from build123d import *

# Parameters (mm, degrees)
SKETCH1_W           = 4
SKETCH1_H           = 15
BOSS_EXTRUDE1_DEPTH = 4
SKETCH2_R           = 0.925
BOSS_EXTRUDE2_DEPTH = 2
BOSS_EXTRUDE3_DEPTH = 2
SKETCH6_W           = 5
SKETCH6_H           = 5
BOSS_EXTRUDE5_DEPTH = 7.5
SKETCH7_R           = 0.925
BOSS_EXTRUDE6_DEPTH = 18
CHAMFER1_SIZE       = 0.5


with BuildPart() as part:
    # Sketch1 → Boss-Extrude1 (new body)
    with BuildSketch(Plane(origin=(0, 0, 0), x_dir=(1, 0, 0), z_dir=(0, 1, 0))):
        Rectangle(SKETCH1_W, SKETCH1_H)
    extrude(amount=BOSS_EXTRUDE1_DEPTH)

    # Sketch2 → Boss-Extrude2 (add)
    with BuildSketch(Plane.XY.offset(7.5)):
        with Locations((0, 2)):
            Circle(SKETCH2_R)
    extrude(amount=BOSS_EXTRUDE2_DEPTH)

    # Sketch3 → Boss-Extrude3 (add)
    with BuildSketch(Plane.XY.offset(9.5)):
        with BuildLine():
            Line((-0.75, 2.925), (0.75, 2.925))
            ThreePointArc((0.75, 2.925), (1.675, 2), (0.75, 1.075))
            Line((0.75, 1.075), (-0.75, 1.075))
            ThreePointArc((-0.75, 1.075), (-1.675, 2), (-0.75, 2.925))
        make_face()
    extrude(amount=BOSS_EXTRUDE3_DEPTH)

    # Sketch6 → Boss-Extrude5 (add)
    with BuildSketch(Plane.XY):
        with Locations((0.5, 2.5)):
            Rectangle(SKETCH6_W, SKETCH6_H)
    extrude(amount=-BOSS_EXTRUDE5_DEPTH)

    # Sketch7 → Boss-Extrude6 (add)
    with BuildSketch(Plane.XY.offset(7.5)):
        with Locations((1, 2.832903413)):
            Circle(SKETCH7_R)
    extrude(amount=-BOSS_EXTRUDE6_DEPTH)

    # Chamfer1
    chamfer1_edges = [part.edges().sort_by_distance(p)[0] for p in [
        (-2, 4, 3.75),
        (3, 0, -3.75),
        (-2, 5, -3.75),
        (3, 5, -3.75),
        (2, 4, 3.75),
        (-2, 0, 0),
        (2, 0, 3.75),
    ]]
    chamfer(chamfer1_edges, length=CHAMFER1_SIZE)


solid = part.part
Verification items for the finished model (mm, model axes). A direction names the side the tool comes from. Coordinates: 2 decimals unless noted, no trailing zeros. Order: outer loops, then holes, each group sorted by start corner. A loop starts at its lowest first (then second) coordinate and runs counter-clockwise, first axis right, second up. Notation, with made-up numbers: M 4.25,-3.75 L 21.25,-3.75 A21 ccw 21.25,4.25 Z; hole C 72,49.25 d6. An arc over 180 degrees is marked long. One line per item, written item: value. Start each with the question number.
Item 1: Sectioned sample at B-B (x = 1.25). Enter the section's corners in (y, z), then the cut area to 3 significant figures.
Item 2: Sectioned sample at D-D (y = 1.35). Enter the section's corners in (x, z).
Item 3: Scan lines: probe 1 along Z at (x, y) = (1.05, 2.65); probe 2 along Y at (x, z) = (-0.45, 7.25); probe 3 along Z at (x, y) = (0.65, 0.75). Record each from-to range of solid material in increasing order.
Item 4: Mould release check, pull along Z, two halves, no side actions. Record for faces 5 (the flat face through (0, 2, -7.5)), 6 (the flat face through (0, 1.075, 10)), 7 (the flat face through (-1.2, 2, 9.5)): released by +Z, released by -Z, zero draft, split by the parting line, or undercut.
Item 5: Gauge pin test, flat ends, axial feed: pin 1 (1.6 mm diameter, centred on x = 0, z = 10.5, fed in from +Y) (3 decimals); pin 2 (0.8 mm diameter, centred on x = -1, y = 2, fed in from -Z); pin 3 (0.9 mm diameter, centred on x = 0, z = 4.5, fed in from +Y). Record the tip position at first contact, or that the pin passes through.
Item 6: Sectioned sample at C-C (x = 2.25). Enter the section's corners in (y, z).
Item 7: Sectioned sample at A-A (z = -2.5). Enter the section's corners in (x, y).
Item 8: Access from +Z, -Z, +X, -X, +Y, -Y to the whole of each face (thin tool, end or side, straight path). Record for faces 1 (the flat face through (2, 2, 4)), 2 (the flat face through (0, 2.925, 10)), 3 (the cylindrical face through (1.675, 2.02, 10.486)), 4 (the cylindrical face through (-1.675, 1.98, 10.486)).
Conclusion:
1. outline: M 0,-7.5 L 1.94,-7.5 L 1.94,-10.5 L 3.72,-10.5 L 3.72,-7.5 L 5,-7.5 L 5,0 L 4,0 L 4,7.5 L 0,7.5 Z; M 1.22,9.5 L 2.78,9.5 L 2.78,11.5 L 1.22,11.5 Z
1. area: 76.0 mm^2
2. outline: M -2,-7.5 L 3,-7.5 L 3,0 L 2,0 L 2,7.5 L 0.66,7.5 L 0.66,9.5 L 1.41,9.5 L 1.41,11.5 L -1.41,11.5 L -1.41,9.5 L -0.66,9.5 L -0.66,7.5 L -2,7.5 Z
3. probe 1: z = -10.5 to 7.5, 9.5 to 11.5
3. probe 2: y = 0 to 4
3. probe 3: z = -7.5 to 7.5
4. face 5: released by -Z
4. face 6: zero draft
4. face 7: undercut
5. pin 1: stops at y = 2.925
5. pin 2: stops at z = -7.5
5. pin 3: stops at y = 4
6. outline: M 0,-7.5 L 5,-7.5 L 5,0 L 0,0 Z
7. outline: M -2,0.5 L -1.5,0 L 2.5,0 L 3,0.5 L 3,4.5 L 2.5,5 L -1.5,5 L -2,4.5 Z
8. face 1: +Z, +X, +Y, -Y
8. face 2: +Z, +X, -X, +Y
8. face 3: +Z, +X
8. face 4: +Z, -X
